Model file for the job. Use its own axes, mm. Round coordinates to 2 decimals unless told otherwise and drop trailing zeros. Order: outer loops, then holes, each group sorted by start corner. A loop starts at its lowest first (then second) coordinate and runs counter-clockwise, first axis right, second up. Notation, with made-up numbers: (6.5, 56.25) - (25.5, 56.25) arc R23 cw to (25.5, 69.25) - close; hole circle Ø10 at (43.5, 46.5). An arc over 180 degrees is marked (long way). Answer as CSV lines item,"result". Start each with the question number.
1. Band-saw the part on D-D on x = 0. List the corners of the cut face in (y, z), then the cut area to 3 significant figures.
2. Pin check, flat tips, straight feed: pin 1 Ø0.7 at (y, z) = (0.5, -11.5) entering from +X; pin 2 Ø0.7 at (y, z) = (0, -16.5) entering from -X; pin 3 Ø0.7 at (y, z) = (-2, -27) entering from -X. Stop position of each tip, or through.
3. Band-saw the part on B-B on z = -32.5. List the corners of the cut face in (x, y).
4. Band-saw the part on C-C on y = 0. List the corners of the cut face in (x, z), then the cut area to 3 significant figures.
5. Band-saw the part on A-A on y = 2.75. List the corners of the cut face in (x, z), then the cut area to 3 significant figures.
6. Wall check: line 1 along X through (y, z) = (-2, -32.5); line 2 along X through (y, z) = (0.25, -6.5); line 3 along Y through (x, z) = (0.1, -12). Give the ranges that are in metal, low to high. Write a range as [from, to].
```python
from build123d import *

# Parameters (mm, degrees)
EXTRUDE_1_DEPTH = 45
FILLET_1_R      = 0.1


with BuildPart() as part:
    # 草图1 → 凸台-拉伸1 (new body)
    with BuildSketch(Plane.XY):
        with BuildLine():
            Line((-1.95, -2.5), (-0.5, -2.5))
            Line((-0.5, -2.5), (-0.5, -1))
            Line((-0.5, -1), (0.5, -1))
            Line((0.5, -1), (0.5, -2.5))
            Line((0.5, -2.5), (1.95, -2.5))
            Line((1.95, -2.5), (1.95, -1.555590279))
            ThreePointArc((1.95, -1.555590279), (1.780042303, -1.088161527), (1.5, -0.677124344))
            Line((1.5, -0.677124344), (1.5, 0.677124344))
            ThreePointArc((1.5, 0.677124344), (1.912032648, 2.586626929), (0.5, 3.936491673))
            Line((0.5, 3.936491673), (0.5, 0.936491673))
            Line((0.5, 0.936491673), (-0.5, 0.936491673))
            Line((-0.5, 0.936491673), (-0.5, 3.936491673))
            ThreePointArc((-0.5, 3.936491673), (-1.912032648, 2.586626929), (-1.5, 0.677124344))
            Line((-1.5, 0.677124344), (-1.5, -0.677124344))
            ThreePointArc((-1.5, -0.677124344), (-1.780042303, -1.088161527), (-1.95, -1.555590279))
            Line((-1.95, -1.555590279), (-1.95, -2.5))
        make_face()
    extrude(amount=-EXTRUDE_1_DEPTH)

    # 圆角1
    fillet_1_edges = [part.edges().sort_by_distance(p)[0] for p in [
        (1.95, -2.5, -22.5),
        (-1.95, -2.5, -22.5),
    ]]
    fillet(fillet_1_edges, radius=FILLET_1_R)


solid = part.part
```
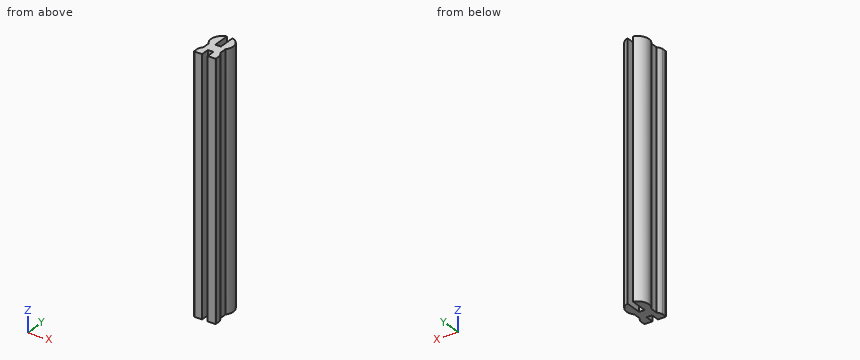
Reply:
1,outline,"(-1, -45) - (0.94, -45) - (0.94, 0) - (-1, 0) - close"
1,area,"87.1 mm2"
2,pin 1,"stops at x = 1.64"
2,pin 2,"stops at x = -1.5"
2,pin 3,"stops at x = -1.95"
3,outline,"(-1.95, -2.4) arc R0.1 ccw to (-1.85, -2.5) - (-0.5, -2.5) - (-0.5, -1) - (0.5, -1) - (0.5, -2.5) - (1.85, -2.5) arc R0.1 ccw to (1.95, -2.4) - (1.95, -1.56) arc R2 ccw to (1.5, -0.68) - (1.5, 0.68) arc R2 ccw to (0.5, 3.94) - (0.5, 0.94) - (-0.5, 0.94) - (-0.5, 3.94) arc R2 ccw to (-1.5, 0.68) - (-1.5, -0.68) arc R2 ccw to (-1.95, -1.56) - close"
4,outline,"(-1.5, -45) - (1.5, -45) - (1.5, 0) - (-1.5, 0) - close"
4,area,"135 mm2"
5,outline,"(-1.85, -45) - (-0.5, -45) - (-0.5, 0) - (-1.85, 0) - close; (0.5, -45) - (1.85, -45) - (1.85, 0) - (0.5, 0) - close"
5,area,"122 mm2"
6,line 1,"x = [-1.95, -0.5], [0.5, 1.95]"
6,line 2,"x = [-1.5, 1.5]"
6,line 3,"y = [-1, 0.94]"
